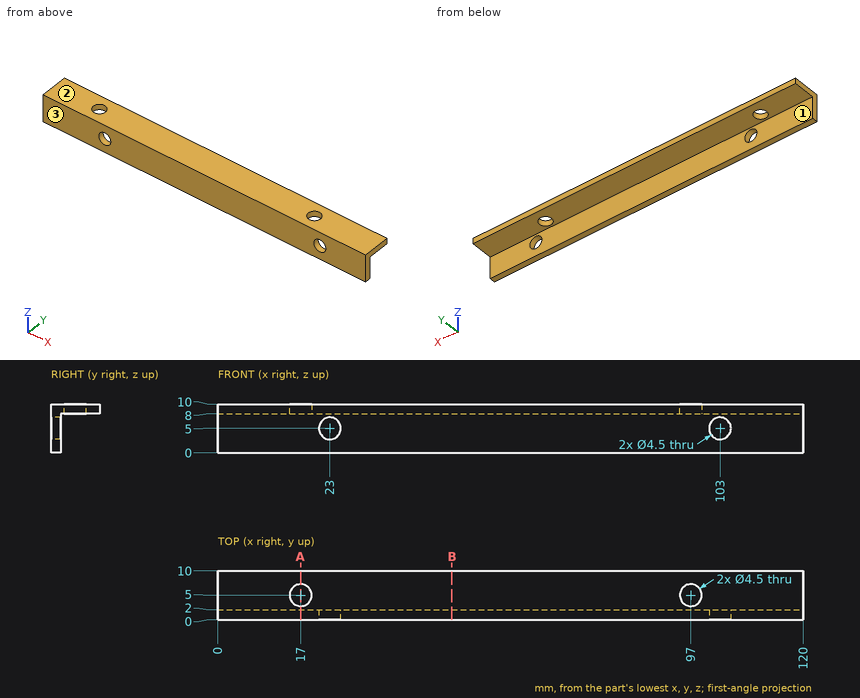
Design review of the part shown in the three views and the two pictorial views. Dimensions are in mm from the part's minimum x, y and z. Coordinates: 2 decimals unless noted, no trailing zeros. Order: outer loops, then holes, each group sorted by start corner. A loop starts at its lowest first (then second) coordinate and runs counter-clockwise, first axis right, second up. Notation, with made-up numbers: (56, -29.5) - (96, -29.5) arc R21 ccw to (96, -5.5) - close; hole circle Ø9 at (4.5, 64). An arc over 180 degrees is marked (long way). One line per question, with ' | ' between items.
Q1. The part is to be moulded in two halves that separate along Y. For the marked faces 1, 2 and 3, say which applies: +Y half, -Y half, draft (parallel to the pull), parting line (faces both ways), or undercut.
Answer key:
face 1: +Y half | face 2: draft | face 3: -Y half
Q2. Consider section A-A, the plane x = 17. Give the boundary of the cut face in (y, z).
Answer key:
outline: (0, 0) - (2, 0) - (2, 8) - (2.75, 8) - (2.75, 10) - (0, 10) - close; (7.25, 8) - (10, 8) - (10, 10) - (7.25, 10) - close
Q3. Consider section B-B, the plane x = 48. Give the boundary of the cut face in (y, z), then the cut area to 3 significant figures.
Answer key:
outline: (0, 0) - (2, 0) - (2, 8) - (10, 8) - (10, 10) - (0, 10) - close | area: 36.0 mm2
Q4. Clearance check with flat-ended pins moving along their axes: pin 1 Ø2.5 at (x, z) = (53.5, 6) entering from +Y; pin 2 Ø3 at (x, y) = (26.5, 7.5) entering from -Z. State where each tip first meets the part, or that it passes through.
Answer key:
pin 1: stops at y = 2 | pin 2: stops at z = 8
Q5. To check wall thickness, follow line 1 along Y through (x, z) = (97, 9); line 2 along X through (y, z) = (1.5, 4.25). State the ranges of each line that lie inside material, in increasing order.
Answer key:
line 1: y = 0 to 2.75, 7.25 to 10 | line 2: x = 0 to 20.88, 25.12 to 100.88, 105.12 to 120
